Print and shaded views of the part. All mm, measured from the part's lowest x, y and z. A direction names the side the tool comes from. Round coordinates to 2 decimals unless told otherwise and drop trailing zeros. Write each loop counter-clockwise with the first axis right and the second up, starting at its lowest first coordinate (ties: lowest second). Pieces come first, ordered by that corner, then holes. Notation, with made-up numbers: (44.5, 51) - (49.5, 51) arc R12 cw to (49.5, 60) - close; hole circle Ø9 at (81.5, 40.5). An arc over 180 degrees is marked (long way). Put each result on its own line as item: value. Start each with the question number.
Item 1: Cut at C-C (y = 3.25). Give the cut face in (x, z).
Item 2: Drill centre lines: line 1 (X direction, y = 8.5, z = 17.5); line 2 (X direction, y = 11, z = 17.5); line 3 (X direction, y = 2.75, z = 18). Where is each one in solid material? Low to high. Write a range as from..to.
Item 3: Cut at B-B (x = 17.5). Give the cut face in (y, z), and give its area (3 significant figures).
Item 4: 3-axis set-ups, long thin cutter, end or side, ignore diameter. For the marked faces 1 and 2: which of +Z, -Z, +X, -X, +Y, -Y reach the whole face in a straight line?
Item 5: Pin check, flat tips, straight feed: pin 1 Ø8 at (x, z) = (25, 18) entering from -Y; pin 2 Ø5 at (y, z) = (5.5, 5.5) entering from +X. Stop position of each tip, or through.
Item 6: Cut at A-A (z = 17.5). Give the cut face in (x, y), and give its area (3 significant figures).
Item 7: Cut at D-D (y = 12). Give the cut face in (x, z).
Item 8: Mould opens along Z. For the marked faces 3, 4 and 5 say: released by +Z, released by -Z, zero draft, split by the parting line, or undercut.
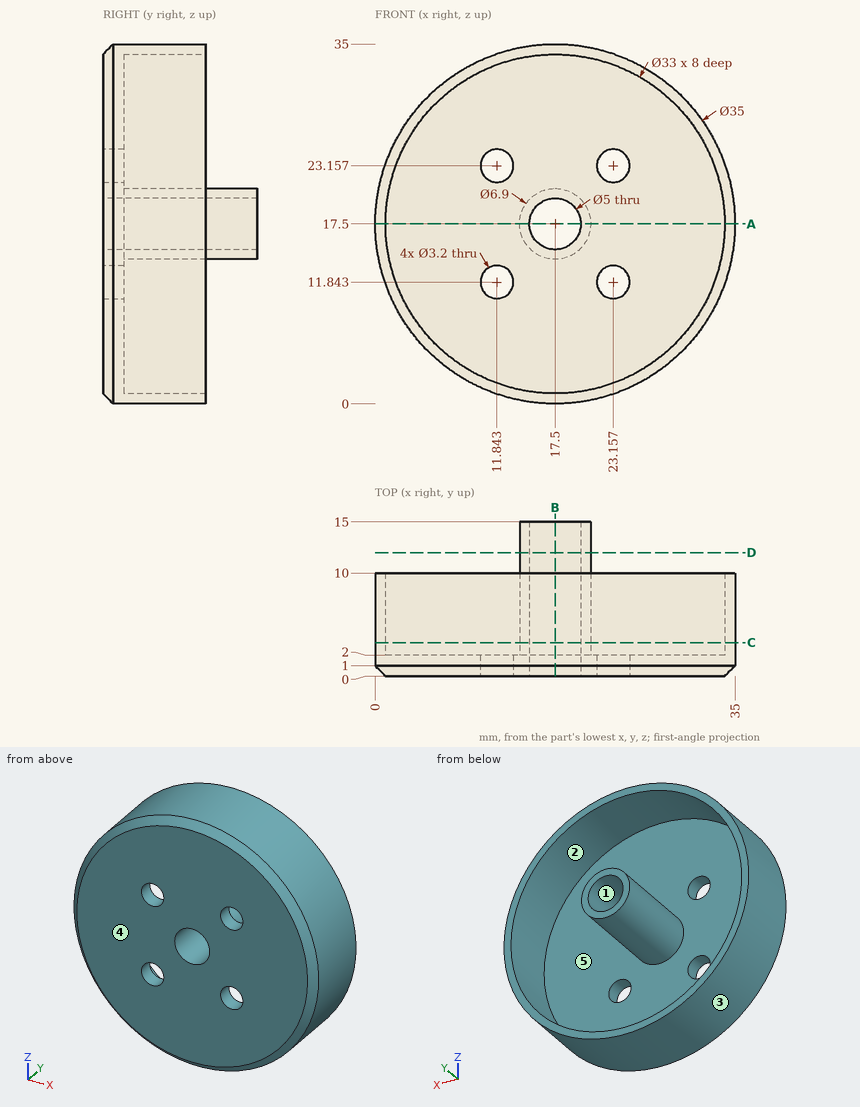
Output values:
1. outline: circle Ø35 at (17.5, 17.5); circle Ø6.9 at (17.5, 17.5); hole circle Ø33 at (17.5, 17.5); hole circle Ø5 at (17.5, 17.5)
2. line 1: 0..1, 14.05..15, 20..20.95, 34..35
2. line 2: 14.05..15, 20..20.95
2. line 3: 0.01..1.01, 14.09..15.05, 19.95..20.91, 33.99..34.99
3. outline: (0, 1) - (1, 0) - (10, 0) - (10, 1) - (2, 1) - (2, 14.05) - (15, 14.05) - (15, 15) - (0, 15) - close; (0, 20) - (15, 20) - (15, 20.95) - (2, 20.95) - (2, 34) - (10, 34) - (10, 35) - (1, 35) - (0, 34) - close
3. area: 99.7 mm2
4. face 1: +Y, -Y
4. face 2: +Y
5. pin 1: y = 0
5. pin 2: x = 32.2
6. outline: (0, 1) - (1, 0) - (15, 0) - (15, 15) - (14.05, 15) - (14.05, 2) - (1, 2) - (1, 10) - (0, 10) - close; (20, 0) - (34, 0) - (35, 1) - (35, 10) - (34, 10) - (34, 2) - (20.95, 2) - (20.95, 15) - (20, 15) - close
6. area: 99.7 mm2
7. outline: circle Ø6.9 at (17.5, 17.5); hole circle Ø5 at (17.5, 17.5)
8. face 3: split by the parting line
8. face 4: zero draft
8. face 5: undercut
